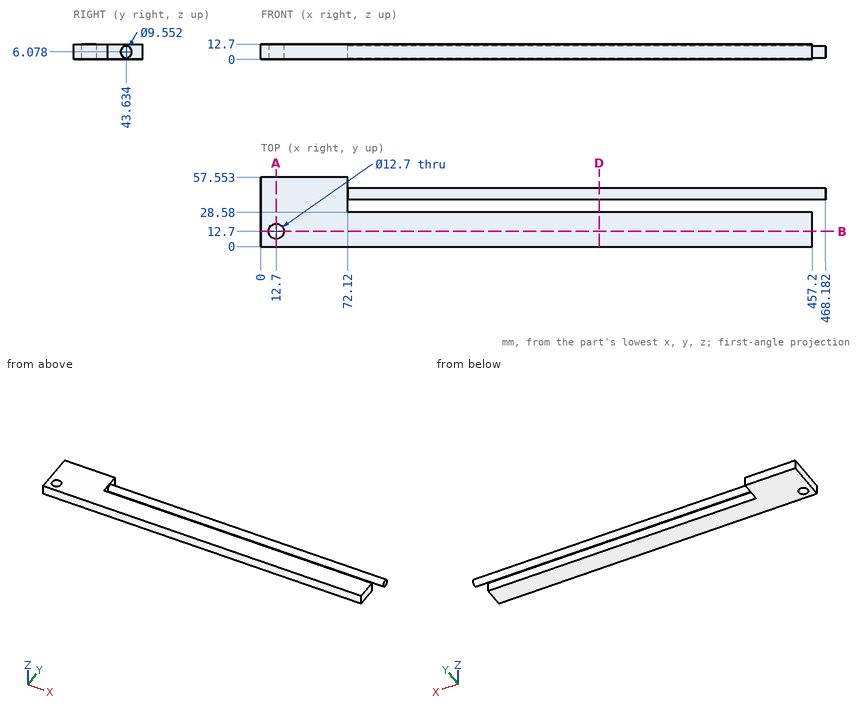
Here's the drawing with two shaded views (mm, measured from the low corner). I have some questions. Coordinates: 2 decimals unless noted, no trailing zeros. Order: outer loops, then holes, each group sorted by start corner. A loop starts at its lowest first (then second) coordinate and runs counter-clockwise, first axis right, second up. Notation, with made-up numbers: (-14.5, -0.75) - (22.5, -0.75) arc R29 cw to (22.5, 37.25) - close; hole circle Ø11 at (83.25, 30). An arc over 180 degrees is marked (long way). Use CSV: the item, a comma, the result in double quotes. Start each with the question number.
1. Please list where these lines run through material, in increasing order: line 1 (Y direction, x = 12.7, z = 5.75); line 2 (X direction, y = 12.7, z = 6.25); line 3 (X direction, y = 5, z = 9.75). Write a range as from..to.
2. I'm going to push flat-ended pins straight in: pin 1 (3 mm diameter, centred on y = 45.5, z = 11, fed in from +X); pin 2 (5 mm diameter, centred on x = 196.5, z = 4.5, fed in from +Y); pin 3 (1 mm diameter, centred on y = 52, z = 2.5, fed in from +X). Where does each tip first touch, or does it pass through?
3. Suppose I cut it at A-A on x = 12.7. List the corners of the cut face in (y, z) for me, then the cut area to 3 significant figures.
4. Suppose I cut it at D-D on x = 280.5. List the corners of the cut face in (y, z) for me (1 decimal), then the cut area to 3 significant figures.
5. Suppose I cut it at B-B on y = 12.7. List the corners of the cut face in (x, z) for me.
Output:
1,line 1,"y = 0..6.35, 19.05..57.55"
1,line 2,"x = 0..6.35, 19.05..457.2"
1,line 3,"x = 0..457.2"
2,pin 1,"stops at x = 468.18"
2,pin 2,"stops at y = 48.41"
2,pin 3,"stops at x = 72.12"
3,outline,"(0, 0) - (6.35, 0) - (6.35, 12.7) - (0, 12.7) - close; (19.05, 0) - (57.55, 0) - (57.55, 12.7) - (19.05, 12.7) - close"
3,area,"570 mm2"
4,outline,"(0, 0) - (28.6, 0) - (28.6, 12.7) - (0, 12.7) - close; circle Ø9.6 at (43.6, 6.1)"
4,area,"435 mm2"
5,outline,"(0, 0) - (6.35, 0) - (6.35, 12.7) - (0, 12.7) - close; (19.05, 0) - (457.2, 0) - (457.2, 12.7) - (19.05, 12.7) - close"
